```python
from build123d import *

# Parameters (mm, degrees)
F0_W     = 38
F0_H     = 21.5
F1_DEPTH = 3
F2_W     = 38
F2_H     = 3
F3_DEPTH = 55
F4_R     = 2.5
F5_DEPTH = 21.501


with BuildPart() as f1:
    # F0 (on Front) → F1 (new body)
    with BuildSketch(Plane.XZ):
        Rectangle(F0_W, F0_H)
        with BuildLine():
            ThreePointArc((-14, -8), (-16.75, -5.25), (-14, -2.5))
            Line((-14, -2.5), (-6, -2.5))
            ThreePointArc((-6, -2.5), (-3.25, -5.25), (-6, -8))
            Line((-6, -8), (-14, -8))
        make_face(mode=Mode.SUBTRACT)
        with BuildLine():
            Line((14, -8), (6, -8))
            ThreePointArc((6, -8), (3.25, -5.25), (6, -2.5))
            Line((6, -2.5), (14, -2.5))
            ThreePointArc((14, -2.5), (16.75, -5.25), (14, -8))
        make_face(mode=Mode.SUBTRACT)
    extrude(amount=F1_DEPTH)

    # F2 (on face) → F3 (join)
    with BuildSketch(Plane.XZ.offset(3)):
        with Locations((0, 9.25)):
            Rectangle(F2_W, F2_H)
    extrude(amount=-F3_DEPTH)

    # F4 (on face) → F5 (cut, through all)
    with BuildSketch(Plane.XY.offset(10.75)):
        with Locations((0, 10.5)):
            Circle(F4_R)
    extrude(amount=-F5_DEPTH, mode=Mode.SUBTRACT)


solid = f1.part
```
Verification items for the finished model (mm, model axes). A direction names the side the tool comes from. Coordinates: 2 decimals unless noted, no trailing zeros. Write each loop counter-clockwise with the first axis right and the second up, starting at its lowest first coordinate (ties: lowest second). Pieces come first, ordered by that corner, then holes. Notation, with made-up numbers: M -15,-19.75 L 5,-19.75 A15 cw 5,-5.75 Z; hole C 2,85.5 d8. An arc over 180 degrees is marked long. Answer as a JSON object with one key per item and string values. Group by question number.
(1) Material ranges on line 1 (Y direction, x = 0, z = 9.85); line 2 (Z direction, x = -1.5, y = 14.5); line 3 (Y direction, x = 5, z = 5.25), recorded low to high.
(2) Release check for a two-part mould opening along Z. For faces 4 (the face through (0, 25, 10.75)), 5 (the face through (0, 0, 1)), 6 (the face through (-10, -1, -8)) record: +Z half, -Z half, draft (parallel to the pull), parting line (faces both ways), or undercut.
(3) Tool access check on faces 1 (the face through (0, 26, 7.75)), 2 (the face through (16.75, -1.48, -5.19)), 3 (the face through (-0.54, 8.06, 9.27)). Record the directions out of +Z, -Z, +X, -X, +Y, -Y that give a thin tool (end or side, any length) a straight path to the whole face; none if there is none.
(4) Cross-section at C-C, the plane z = -5.25. Record the cut outline in (x, y).
(5) Cross-section at D-D, the plane x = -1.5. Record the cut outline in (y, z), and give its area (4 significant figures).
(6) Cross-section at B-B, the plane y = 10.5. Record the cut outline in (x, z).
(7) Cross-section at A-A, the plane x = -11. Record the cut outline in (y, z), and give its area (3 significant figures).
(8) Gauge pin test, flat ends, axial feed: pin 1 (10 mm diameter, centred on x = 5, z = -4.5, fed in from +Y); pin 2 (8 mm diameter, centred on x = -1, y = 22.5, fed in from -Z). Record the tip position at first contact, or that the pin passes through.
Reply:
{
 "1": {"line 1": "-3 to 8, 13 to 52", "line 2": "7.75 to 10.75", "line 3": "-3 to 0"},
 "2": {"face 4": "+Z half", "face 5": "draft", "face 6": "undercut"},
 "3": {"face 1": "-Z, +X, -X, +Y", "face 2": "+Y, -Y", "face 3": "+Z, -Z"},
 "4": {"outline": "M -19,-3 L -16.75,-3 L -16.75,0 L -19,0 Z; M -3.25,-3 L 3.25,-3 L 3.25,0 L -3.25,0 Z; M 16.75,-3 L 19,-3 L 19,0 L 16.75,0 Z"},
 "5": {"outline": "M -3,-10.75 L 0,-10.75 L 0,7.75 L 8.5,7.75 L 8.5,10.75 L -3,10.75 Z; M 12.5,7.75 L 52,7.75 L 52,10.75 L 12.5,10.75 Z", "area": "208.5 mm²"},
 "6": {"outline": "M -19,7.75 L -2.5,7.75 L -2.5,10.75 L -19,10.75 Z; M 2.5,7.75 L 19,7.75 L 19,10.75 L 2.5,10.75 Z"},
 "7": {"outline": "M -3,-10.75 L 0,-10.75 L 0,-8 L -3,-8 Z; M -3,-2.5 L 0,-2.5 L 0,7.75 L 52,7.75 L 52,10.75 L -3,10.75 Z", "area": "204 mm²"},
 "8": {"pin 1": "y = 0", "pin 2": "z = 7.75"}
}
